Work out the finished part from the listing and answer in its coordinate system (mm). Coordinates: 2 decimals unless noted, no trailing zeros. Order: outer loops, then holes, each group sorted by start corner. A loop starts at its lowest first (then second) coordinate and runs counter-clockwise, first axis right, second up. Notation, with made-up numbers: M 82,17 L 89,17 A20 cw 89,51 Z; hole C 33,45 d5. An arc over 180 degrees is marked long. Write item = value, one per line. Start each with the question number.
Q1. Find section B-B on x = -1712.5. Give the vertices of the cut face in (y, z).
Q2. Find section C-C on y = -9. Give the vertices of the cut face in (x, z).
Q3. Straight lines are drawn through the part: line 1 along X through (y, z) = (28, 1.2); line 2 along X through (y, z) = (24, 2.25); line 3 along X through (y, z) = (30, 1.1). For each, find the intervals that lie inside material, in ascending order.
Q4. Find section D-D on y = 17. Give the vertices of the cut face in (x, z), and give its area (3 significant figures).
Q5. Find section A-A on z = 0.55. Give the vertices of the cut face in (x, y), and give its area (3 significant figures).
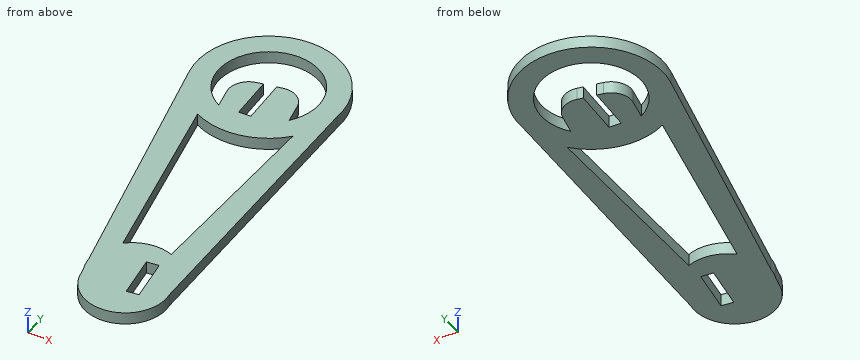
```python
from build123d import *

# Parameters (mm, degrees)
BASE_EXTRUDE_DEPTH = 3
CUT_EXTRUDE2_DEPTH = 98
CUT_EXTRUDE6_DEPTH = 32


with BuildPart() as part:
    # Sketch1 → Base-Extrude (new body)
    with BuildSketch(Plane.XY):
        with BuildLine():
            Line((-1733.906004377, 29.697699618), (-1717.660054383, -37.356142617))
            ThreePointArc((-1717.660054383, -37.356142617), (-1717.392491193, -39.067926894), (-1716.846904921, -40.712351137))
            Line((-1716.846904921, -40.712351137), (-1716.417156793, -42.486101711))
            ThreePointArc((-1716.417156793, -42.486101711), (-1704.630486547, -50.750700002), (-1696.365888256, -38.964029756))
            Line((-1696.365888256, -38.964029756), (-1698.635055574, 32.835792941))
            ThreePointArc((-1698.635055574, 32.835792941), (-1718.097908318, 51.805768332), (-1733.906004377, 29.697699618))
        make_face()
        with BuildLine():
            Line((-1703.09668856, 22.095884858), (-1703.438627674, -26.79881214))
            ThreePointArc((-1703.438627674, -26.79881214), (-1709.186992556, -26.294688909), (-1714.332729754, -28.906054021))
            Line((-1714.332729754, -28.906054021), (-1724.517294461, 17.943098305))
            ThreePointArc((-1724.517294461, 17.943098305), (-1713.101655099, 16.381275869), (-1703.09668856, 22.095884858))
        make_face(mode=Mode.SUBTRACT)
        with BuildLine():
            Line((-1719.582465885, 33.977627673), (-1713.717650395, 35.244094915))
            ThreePointArc((-1713.717650395, 35.244094915), (-1709.952658337, 34.558897322), (-1707.774914786, 31.412138042))
            Line((-1707.774914786, 31.412138042), (-1706.689581956, 26.386128223))
            ThreePointArc((-1706.689581956, 26.386128223), (-1719.129096181, 46.090906116), (-1722.329089928, 23.008882245))
            Line((-1722.329089928, 23.008882245), (-1723.414422758, 28.034892064))
            ThreePointArc((-1723.414422758, 28.034892064), (-1722.729225165, 31.799884122), (-1719.582465885, 33.977627673))
        make_face(mode=Mode.SUBTRACT)
    extrude(amount=BASE_EXTRUDE_DEPTH)

    # Sketch2 → Cut-Extrude2 (cut)
    with BuildSketch(Plane.XY.offset(3)):
        Polygon((-1715.450740146, 40.629639019), (-1714.419013149, 23.325108151), (-1717.413695187, 23.146559866), (-1718.008856137, 33.128833327), (-1718.445422184, 40.451090735), align=None)
    extrude(amount=-CUT_EXTRUDE2_DEPTH, mode=Mode.SUBTRACT)

    # Sketch4 → Cut-Extrude6 (cut)
    with BuildSketch(Plane(origin=(0, 0, 0), x_dir=(-1, 0, 0), z_dir=(0, 0, -1))):
        Polygon((1704.858484276, -42.808076116), (1706.594681007, -31.821068487), (1703.587915488, -31.424502176), (1701.889253436, -42.379510814), align=None)
    extrude(amount=-CUT_EXTRUDE6_DEPTH, mode=Mode.SUBTRACT)


solid = part.part
```
Findings below:
q1.outline = M -48.87,0 L -27.54,0 L -27.54,3 L -48.87,3 Z; M 16.51,0 L 35.35,0 L 35.35,3 L 16.51,3 Z; M 45.7,0 L 51.42,0 L 51.42,3 L 45.7,3 Z
q2.outline = M -1724.53,0 L -1718.66,0 L -1718.66,3 L -1724.53,3 Z; M -1703.31,0 L -1697.31,0 L -1697.31,3 L -1703.31,3 Z
q3.line_1 = -1733.49 to -1727.39, -1723.41 to -1717.7, -1714.7 to -1707.04, -1705.63 to -1698.48
q3.line_2 = -1732.53 to -1723.9, -1722.54 to -1717.46, -1714.46 to -1698.36
q3.line_3 = -1733.98 to -1728.27, -1723.44 to -1717.82, -1714.82 to -1707.47, -1704.76 to -1698.55
q4.outline = M -1730.83,0 L -1724.31,0 L -1724.31,3 L -1730.83,3 Z; M -1722.25,0 L -1710.77,0 L -1710.77,3 L -1722.25,3 Z; M -1703.13,0 L -1698.13,0 L -1698.13,3 L -1703.13,3 Z
q4.area = 69.0 mm^2
q5.outline = M -1733.91,29.7 L -1717.66,-37.36 A10.49 ccw -1716.85,-40.71 L -1716.42,-42.49 A10.18 ccw -1696.37,-38.96 L -1698.64,32.84 A17.91 ccw long Z; hole M -1724.52,17.94 L -1714.33,-28.91 A10.49 cw -1703.44,-26.8 L -1703.1,22.1 A17.91 cw Z; hole M -1723.41,28.03 A5 cw -1719.58,33.98 L -1718.08,34.3 L -1717.41,23.15 L -1714.42,23.33 L -1715.11,34.94 L -1713.72,35.24 A5 cw -1707.77,31.41 L -1706.69,26.39 A12.41 ccw long -1722.33,23.01 Z; hole M -1706.59,-31.82 L -1704.86,-42.81 L -1701.89,-42.38 L -1703.59,-31.42 Z
q5.area = 1,700 mm^2
